Input: part model. Units: mm. Frame: model coordinates. A direction names the side the tool comes from. Give positions to 0.01 mm unless a question says otherwise; leave off trailing zeros. Order: outer loops, then holes, each group sorted by start corner. A loop starts at its lowest first (then second) coordinate and runs counter-clockwise, first axis right, second up. Notation, with made-up numbers: (3, -12.75) - (32, -12.75) arc R22 cw to (32, 11.25) - close; hole circle Ø10 at (-4.75, -24). An arc over 180 degrees is marked (long way). Use a Markdown table: item, result.
Autodesk Inventor part; units mm, degrees
ref_plane "YZ Plane" through (0, 0, 0) normal (1, 0, 0) x (0, 1, 0)
ref_plane "XZ Plane" through (0, 0, 0) normal (0, 1, 0) x (-1, 0, 0)
ref_plane "XY Plane" through (0, 0, 0) normal (0, 0, 1) x (1, 0, 0)
sketch "Sketch1" plane through (0, 0, 0) normal (0, 1, 0) x (-1, 0, 0)
  line L0 (0, 0) -> (10, 0)
  line L1 (10, 0) -> (10, -165)
  line L2 (10, -165) -> (0, -165)
  line L3 (0, -165) -> (0, 0)
  dimension "d0" = 10
  dimension "d1" = 165
extrude "Extrusion1" add sketch "Sketch1" along normal blind 200
sketch "Sketch2" plane through (-10, 0, 0) normal (0, 0, 1) x (1, 0, 0)
  line L0 (2.5, 15) -> (7.5, 15)
  line L1 (7.5, 15) -> (7.5, 185)
  line L2 (7.5, 185) -> (2.5, 185)
  line L3 (2.5, 185) -> (2.5, 15)
  point P0 (10, 0)
  dimension "d4" = 5
  dimension "d5" = 170
extrude "Extrusion2" add sketch "Sketch2" along normal blind 25
sketch "Sketch3" plane through (0, 0, -165) normal (0, 0, -1) x (-1, 0, 0)
  line L0 (2.5, 15) -> (7.5, 15)
  line L1 (7.5, 15) -> (7.5, 185)
  line L2 (7.5, 185) -> (2.5, 185)
  line L3 (2.5, 185) -> (2.5, 15)
  point P0 (0, 0)
  dimension "d8" = 5
  dimension "d9" = 170
extrude "Extrusion3" add sketch "Sketch3" along normal blind 25
sketch "Sketch4" plane through (-10, 0, -165) normal (-1, 0, 0) x (0, 0, 1)
  line L0 (0, 200) -> (165, 200)
  line L1 (82.5, 200) -> (82.5, 0) construction
  line L2 (0, 0) -> (165, 0)
  line L3 (107.5, 175) -> (132.5, 175)
  line L4 (132.5, 175) -> (132.5, 25)
  line L5 (132.5, 25) -> (107.5, 25)
  line L6 (107.5, 25) -> (107.5, 175)
  line L7 (57.5, 175) -> (32.5, 175)
  line L8 (32.5, 175) -> (32.5, 25)
  line L9 (32.5, 25) -> (57.5, 25)
  line L10 (57.5, 25) -> (57.5, 175)
  dimension "d12" = 25
  dimension "d13" = 150
  dimension "d14" = 25
  dimension "d15" = 150
extrude "Extrusion4" cut sketch "Sketch4" against normal blind 10
fillet "Fillet1" radius 12.5 8 edges at (-5, 25, -107.5) (-5, 25, -32.5) (-5, 25, -57.5) (-5, 25, -132.5) (-5, 175, -32.5) (-5, 175, -107.5) (-5, 175, -57.5) (-5, 175, -132.5)
properties part number "TSU_MM_Side_Wall"
1. Set-up query: faces 1 (the face through (-4.93, 28.759, -111.064)), 2 (the face through (-2.5, 99, 12)), 3 (the face through (-7.5, 101, 12)), 4 (the face through (-5, 185, -177)). Return all of +Z, -Z, +X, -X, +Y, -Y with unobstructed straight access to the full face (end or side cutting, diameter ignored); none if empty.
Response:
| item | result |
|---|---|
| face 1 | +X, -X |
| face 2 | +Z, +X, +Y, -Y |
| face 3 | +Z, -X, +Y, -Y |
| face 4 | -Z, +X, -X, +Y |
2. Mould query, pull axis Z, two halves, no side actions, for faces 5 (the face through (-5, 101, 25)), 6 (the face through (-4.93, 28.759, -36.064)), 7 (the face through (-5, 200, -81)). Classes: pulls with the +Z half, pulls with the -Z half, needs draft (parallel to the pull), parting line crosses it, or undercut.
Response:
| item | result |
|---|---|
| face 5 | pulls with the +Z half |
| face 6 | undercut |
| face 7 | needs draft |
3. Pin query (flat end, axial travel): pin 1 (2.5 mm diameter, centred on x = -5.5, z = -177.5, fed in from -Y); pin 2 (5.5 mm diameter, centred on x = -6, z = -172.5, fed in from +Y); pin 3 (20 mm diameter, centred on y = 128, z = 10.5, fed in from -X). Return the tip coordinate at first contact, or that it passes through.
Response:
| item | result |
|---|---|
| pin 1 | stops at y = 15 |
| pin 2 | stops at y = 185 |
| pin 3 | stops at x = -7.5 |
4. Section query D-D (y = 172.5). Return loops of the section in (x, z), then the cut area to 3 significant figures.
Response:
| item | result |
|---|---|
| outline | (-10, -165) - (-7.5, -165) - (-7.5, -190) - (-2.5, -190) - (-2.5, -165) - (0, -165) - (0, -127.5) - (-10, -127.5) - close; (-10, -112.5) - (0, -112.5) - (0, -52.5) - (-10, -52.5) - close; (-10, -37.5) - (0, -37.5) - (0, 0) - (-2.5, 0) - (-2.5, 25) - (-7.5, 25) - (-7.5, 0) - (-10, 0) - close |
| area | 1,600 mm^2 |
5. Section query B-B (x = -4). State how many separate pieces and enclosed holes the cut face has, then the cut area to 3 significant figures.
Response:
| item | result |
|---|---|
| separate pieces | 1 |
| enclosed holes | 2 |
| area | 34,300 mm^2 |
6. Section query A-A (y = 86). Return loops of the section in (x, z), then the cut area to 3 significant figures.
Response:
| item | result |
|---|---|
| outline | (-10, -165) - (-7.5, -165) - (-7.5, -190) - (-2.5, -190) - (-2.5, -165) - (0, -165) - (0, -132.5) - (-10, -132.5) - close; (-10, -107.5) - (0, -107.5) - (0, -57.5) - (-10, -57.5) - close; (-10, -32.5) - (0, -32.5) - (0, 0) - (-2.5, 0) - (-2.5, 25) - (-7.5, 25) - (-7.5, 0) - (-10, 0) - close |
| area | 1,400 mm^2 |
7. Material intervals for line 1 along Z through (x, y) = (-1, 137); line 2 along Z through (x, y) = (-6.25, 100); line 3 along Z through (x, y) = (-0.75, 9.5), sorted ascending.
Response:
| item | result |
|---|---|
| line 1 | z = -165 to -132.5, -107.5 to -57.5, -32.5 to 0 |
| line 2 | z = -190 to -132.5, -107.5 to -57.5, -32.5 to 25 |
| line 3 | z = -165 to 0 |
8. Section query C-C (z = -53). Return loops of the section in (x, y).
Response:
| item | result |
|---|---|
| outline | (-10, 0) - (0, 0) - (0, 27.9) - (-10, 27.9) - close; (-10, 172.1) - (0, 172.1) - (0, 200) - (-10, 200) - close |
